Answer from the drawing. Dimensions are ordinates in mm from the lowest x, y and z of the part. A direction names the side the tool comes from. Round coordinates to 2 decimals unless told otherwise and drop trailing zeros. Loops run counter-clockwise (first coordinate to the right, second up) from the corner with the lowest first, then second, coordinate; pieces in that order, holes last. Notation, with made-up numbers: (61.25, -3.5) - (79.25, -3.5) arc R34 cw to (79.25, 26.5) - close; hole circle Ø10 at (78, -10.5). An arc over 180 degrees is marked (long way). Write item = value, one per line. Start each with the question number.
1) A tool of negligible diameter and unlimited length cuts with its end or side. For the marked faces 1 and 2, from which of +Z, -Z, +X, -X, +Y, -Y can it reach the whole face along a straight path? Write none if from no direction.
2) Section D-D, the plane z = 2.75 is taken. Determine the outline of the cut face in (x, y), and give its area (3 significant figures).
3) Given pin 1 Ø5 at (x, z) = (13.5, 8.5) entering from +Y; pin 2 Ø3 at (y, z) = (8.5, 7.5) entering from -X; pin 3 Ø2 at (x, z) = (7.5, 7.5) entering from +Y; pin 4 Ø2 at (x, z) = (1.5, 7) entering from +Y, each flat-ended and moving along its own axis, determine where each tip first touches the part or whether it passes through.
4) Straight lines are drawn through the part: line 1 along X through (y, z) = (2.75, 7.5); line 2 along Y through (x, z) = (4.75, 10.5); line 3 along Y through (x, z) = (12.5, 4.25). For each, find the intervals that lie inside material, in ascending order.
5) Section A-A, the plane x = 7.5 is taken. Determine the outline of the cut face in (y, z), and give its area (3 significant figures).
6) For a pull along X with two mould halves and no side action, classify the marked faces 3, 4 and 5 as released by +X, released by -X, zero draft, split by the parting line, or undercut.
7) Section B-B, the plane z = 7.5 is taken. Determine the outline of the cut face in (x, y).
8) Section C-C, the plane y = 4.25 is taken. Determine the outline of the cut face in (x, z), and give its area (3 significant figures).
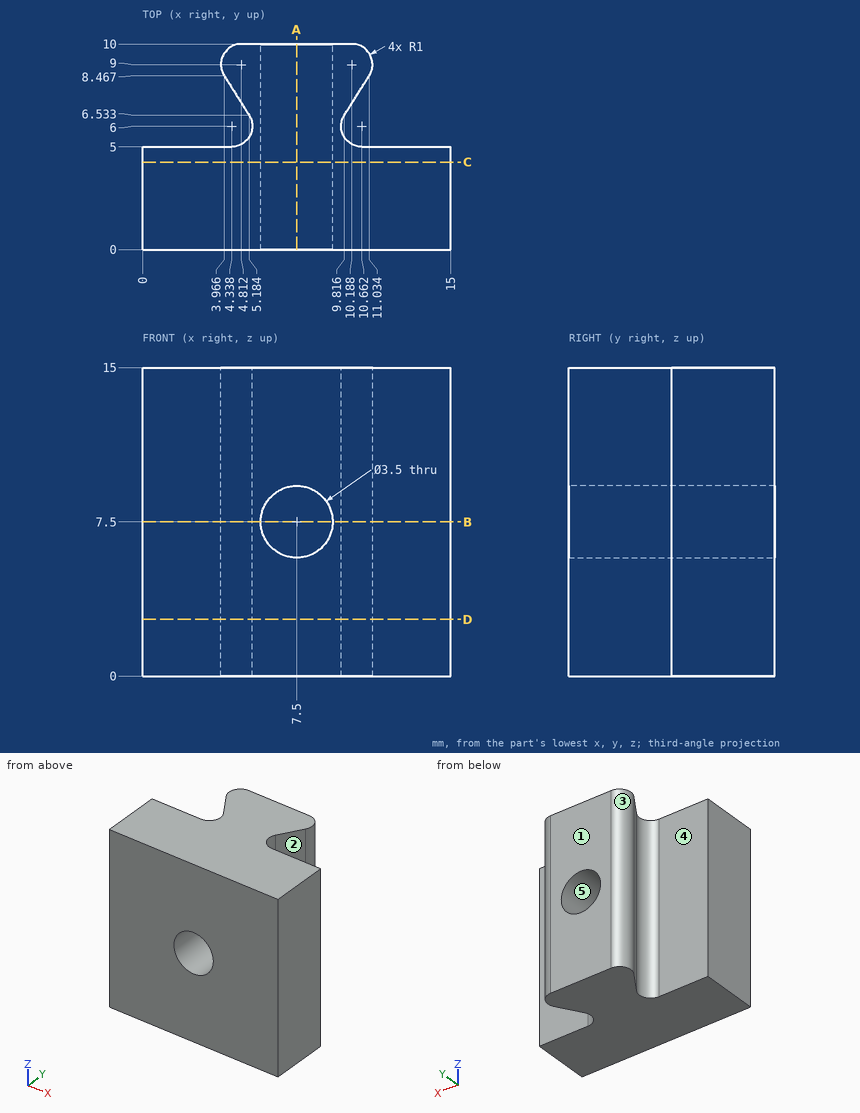
Geometry check:
q1.face_1 = +Z, -Z, +X, -X, +Y
q1.face_2 = +Z, -Z, +X
q2.outline = (0, 0) - (15, 0) - (15, 5) - (10.66, 5) arc R1 cw to (9.82, 6.53) - (11.03, 8.47) arc R1 ccw to (10.19, 10) - (4.81, 10) arc R1 ccw to (3.97, 8.47) - (5.18, 6.53) arc R1 cw to (4.34, 5) - (0, 5) - close
q2.area = 104 mm2
q3.pin_1 = 9.58
q3.pin_2 = 3.81
q3.pin_3 = through
q3.pin_4 = 5
q4.line_1 = 0 to 5.75, 9.25 to 15
q4.line_2 = 0 to 5.09, 7.22 to 10
q4.line_3 = 0 to 5
q5.outline = (0, 0) - (10, 0) - (10, 5.75) - (0, 5.75) - close; (0, 9.25) - (10, 9.25) - (10, 15) - (0, 15) - close
q5.area = 115 mm2
q6.face_3 = released by -X
q6.face_4 = zero draft
q6.face_5 = undercut
q7.outline = (0, 0) - (5.75, 0) - (5.75, 10) - (4.81, 10) arc R1 ccw to (3.97, 8.47) - (5.18, 6.53) arc R1 cw to (4.34, 5) - (0, 5) - close; (9.25, 0) - (15, 0) - (15, 5) - (10.66, 5) arc R1 cw to (9.82, 6.53) - (11.03, 8.47) arc R1 ccw to (10.19, 10) - (9.25, 10) - close
q8.outline = (0, 0) - (15, 0) - (15, 15) - (0, 15) - close; hole circle Ø3.5 at (7.5, 7.5)
q8.area = 215 mm2
